The model under review builds one solid part; all positions refer to its coordinate system, in mm. A direction names the side the tool comes from. Coordinates: 2 decimals unless noted, no trailing zeros. Order: outer loops, then holes, each group sorted by start corner. A loop starts at its lowest first (then second) coordinate and runs counter-clockwise, first axis right, second up. Notation, with made-up numbers: M -28,-33 L 28,-33 A24 ccw 28,-16 Z; hole C -35,78 d1. An arc over 180 degrees is marked long. Answer in a Markdown table with one row per item.
from build123d import *

# Parameters (mm, degrees)
F0_W     = 50.8
F0_H     = 50.8
F1_DEPTH = 2.9718
F2_W     = 5.08
F2_H     = 10.16
F3_DEPTH = 2.9728
F4_W     = 2.2792507852
F4_H     = 2.9790955722
F4_W_2   = 2.794
F4_W_3   = 1.3767347039
F4_H_2   = 2.2981600394
F4_H_3   = 2.7237443884
F4_W_4   = 2.0448682842
F5_DEPTH = 2.9728
F6_W     = 50.8
F6_H     = 2.9718
F7_DEPTH = 25.4
F8_W     = 10.16
F8_H     = 5.08
F8_R     = 1.6637
F9_DEPTH = 2.9718


with BuildPart() as f1:
    # F0 (on Right) → F1 (new body)
    with BuildSketch(Plane.YZ):
        Rectangle(F0_W, F0_H)
    extrude(amount=F1_DEPTH)

    # F2 (on face) → F3 (cut, through all)
    with BuildSketch(Plane.YZ.offset(2.9718)):
        with Locations((-22.86, 7.3814073086)):
            Rectangle(F2_W, F2_H)
        with Locations((-22.86, -6.5885926914)):
            Rectangle(F2_W, F2_H)
    extrude(amount=-F3_DEPTH, mode=Mode.SUBTRACT)

    # F4 (on face) → F5 (cut, through all)
    with BuildSketch(Plane.YZ.offset(2.9718)):
        with Locations((-19.1803746074, 7.6630806953)):
            Rectangle(F4_W, F4_H)
        with Locations((-16.6437492148, 7.6630806953)):
            Rectangle(F4_W_2, F4_H)
        with Locations((-14.5583818629, 7.6630806953)):
            Rectangle(F4_W_3, F4_H)
        with Locations((-16.6437492148, 10.3017085011)):
            Rectangle(F4_W_2, F4_H_2)
        with Locations((-16.6437492148, 4.811660715)):
            Rectangle(F4_W_2, F4_H_3)
        with Locations((-16.8781317158, -3.8333461044)):
            Rectangle(F4_W_2, F4_H_2)
        with Locations((-19.2975658579, -6.4719739102)):
            Rectangle(F4_W_4, F4_H)
        with Locations((-14.7927643638, -6.4719739102)):
            Rectangle(F4_W_3, F4_H)
        with Locations((-16.8781317158, -6.4719739102)):
            Rectangle(F4_W_2, F4_H)
        with Locations((-16.8781317158, -9.3233938905)):
            Rectangle(F4_W_2, F4_H_3)
    extrude(amount=-F5_DEPTH, mode=Mode.SUBTRACT)

    # F6 (on face) → F7 (cut)
    with BuildSketch(Plane.YZ.offset(2.9718)):
        with Locations((0, -23.9141)):
            Rectangle(F6_W, F6_H)
    extrude(amount=-F7_DEPTH, mode=Mode.SUBTRACT)

    # F8 (on face) → F9 (join)
    with BuildSketch(Plane.YZ.offset(2.9718)):
        with Locations((-13.7008163464, -24.9682)):
            Rectangle(F8_W, F8_H)
        with Locations((-13.7008163464, -25.0371717972)):
            Circle(F8_R, mode=Mode.SUBTRACT)
    extrude(amount=-F9_DEPTH)


solid = f1.part
(1) The part is to be moulded in two halves that separate along Z. For faces 4 (the flat face through (0, 0, -1)), 5 (the flat face through (2, -20.32, -10)), 6 (the flat face through (2, 8, -22.428)), 7 (the flat face through (2, -19, 9.153)), say which applies: +Z half, -Z half, draft (parallel to the pull), parting line (faces both ways), or undercut.
Report:
| item | result |
|---|---|
| face 4 | draft |
| face 5 | undercut |
| face 6 | -Z half |
| face 7 | undercut |
(2) Take a section at B-B (y = -0.5). Write out the cut boundary in (x, z).
Report:
| item | result |
|---|---|
| outline | M 0,-22.43 L 2.97,-22.43 L 2.97,25.4 L 0,25.4 Z |
(3) Insertion check: P1, Ø2, axis at y = -13.7, z = -25.04, coming from the +X side; P2, Ø1.6, axis at x = 1, y = -19, coming from the -Z side; P3, Ø1.5, axis at x = 2, z = -6, coming from the -Y side; P4, Ø1.5, axis at x = 1, z = -26, coming from the -Y side. Each pin has a flat end and moves straight along its axis. Give the tip position at first contact, or say it passes through.
Report:
| item | result |
|---|---|
| P1 | through |
| P2 | z = -27.51 |
| P3 | y = -14.1 |
| P4 | y = -18.78 |
(4) Take a section at A-A (z = 4.5). Write out the cut boundary in (x, y), then the cut area to 3 significant figures.
Report:
| item | result |
|---|---|
| outline | M 0,-20.32 L 2.97,-20.32 L 2.97,-18.04 L 0,-18.04 Z; M 0,-15.25 L 2.97,-15.25 L 2.97,25.4 L 0,25.4 Z |
| area | 128 mm^2 |
(5) To check wall thickness, follow line 1 (Z direction, x = 0.2, y = -20); line 2 (Y direction, x = 2.6, z = -3.5); line 3 (Z direction, x = 0.3, y = 2.5). State the ranges of each line that lie inside material, in increasing order. Write a range as [from, to].
Report:
| item | result |
|---|---|
| line 1 | [-22.43, -7.96], [-4.98, 6.17], [9.15, 25.4] |
| line 2 | [-20.32, -18.28], [-15.48, 25.4] |
| line 3 | [-22.43, 25.4] |
(6) Machinability: for faces 1 (the flat face through (2.972, 0, -1)), 2 (the flat face through (2, -20.32, -3)), 3 (the flat face through (2, -15.481, -9)), which of the approach directions +Z, -Z, +X, -X, +Y, -Y give a long, thin tool a straight path to every point of the face, cutting with its end or side? Answer none if there is none.
Report:
| item | result |
|---|---|
| face 1 | +Z, -Z, +X, +Y, -Y |
| face 2 | +X, -X, -Y |
| face 3 | +X, -X |
